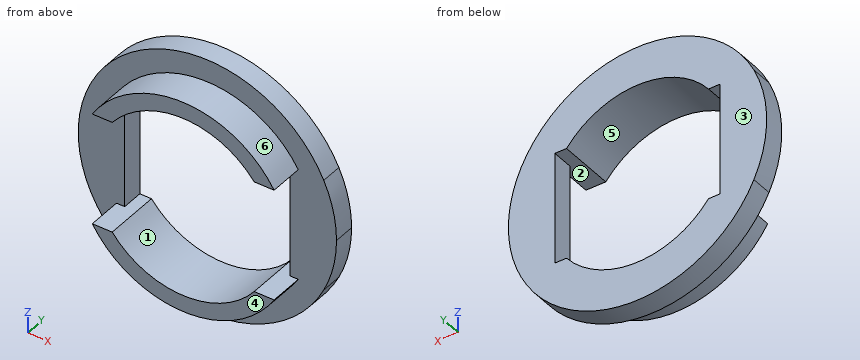
```python
from build123d import *

# Parameters (mm, degrees)
BOSS_EXTRUDE1_DEPTH     = 2.5
BOSS_EXTRUDE2_DEPTH     = 4
CUT_EXTRUDE1_DEPTH      = 5
CUT_EXTRUDE1_DEPTH_BACK = 3.5


with BuildPart() as part:
    # Sketch1 → Boss-Extrude1 (new body)
    with BuildSketch(Plane(origin=(0, 0, 0), x_dir=(1, 0, 0), z_dir=(0, 1, 0))):
        with BuildLine():
            Line((-9.6, -6.5), (-9.6, 6.5))
            Line((-9.6, 6.5), (-13.518505835, 6.5))
            ThreePointArc((-13.518505835, 6.5), (-15, 0), (-13.518505835, -6.5))
            Line((-13.518505835, -6.5), (-9.6, -6.5))
        make_face()
        with BuildLine():
            Line((9.6, -6.5), (-9.6, -6.5))
            Line((-9.6, -6.5), (-13.518505835, -6.5))
            ThreePointArc((-13.518505835, -6.5), (0, -15), (13.518505835, -6.5))
            Line((13.518505835, -6.5), (9.6, -6.5))
        make_face()
        with BuildLine():
            Line((-13.518505835, 6.5), (-9.6, 6.5))
            Line((-9.6, 6.5), (9.6, 6.5))
            Line((9.6, 6.5), (13.518505835, 6.5))
            ThreePointArc((13.518505835, 6.5), (0, 15), (-13.518505835, 6.5))
        make_face()
        with BuildLine():
            Line((13.518505835, 6.5), (9.6, 6.5))
            Line((9.6, 6.5), (9.6, -6.5))
            Line((9.6, -6.5), (13.518505835, -6.5))
            ThreePointArc((13.518505835, -6.5), (14.624937393, -3.333347603), (15, 0))
            ThreePointArc((15, 0), (14.624937393, 3.333347603), (13.518505835, 6.5))
        make_face()
    extrude(amount=BOSS_EXTRUDE1_DEPTH)

    # Sketch2 → Boss-Extrude2 (add)
    with BuildSketch(Plane.XZ):
        with BuildLine():
            ThreePointArc((10.559829544, 6.5), (0, 12.4), (-10.559829544, 6.5))
            Line((-10.559829544, 6.5), (-9.6, 6.5))
            Line((-9.6, 6.5), (-8.246211251, 6.5))
            ThreePointArc((-8.246211251, 6.5), (0, 10.5), (8.246211251, 6.5))
            Line((8.246211251, 6.5), (9.6, 6.5))
            Line((9.6, 6.5), (10.559829544, 6.5))
        make_face()
        with BuildLine():
            Line((-9.6, -6.5), (-10.559829544, -6.5))
            ThreePointArc((-10.559829544, -6.5), (0, -12.4), (10.559829544, -6.5))
            Line((10.559829544, -6.5), (9.6, -6.5))
            Line((9.6, -6.5), (8.246211251, -6.5))
            ThreePointArc((8.246211251, -6.5), (0, -10.5), (-8.246211251, -6.5))
            Line((-8.246211251, -6.5), (-9.6, -6.5))
        make_face()
    extrude(amount=BOSS_EXTRUDE2_DEPTH)

    # Sketch2<3> → Cut-Extrude1 (cut, two sides)
    with BuildSketch(Plane.XZ) as cut_extrude1_sk:
        with BuildLine():
            ThreePointArc((8.246211251, 6.5), (0, 10.5), (-8.246211251, 6.5))
            Line((-8.246211251, 6.5), (8.246211251, 6.5))
        make_face()
        with BuildLine():
            Line((8.246211251, -6.5), (-8.246211251, -6.5))
            ThreePointArc((-8.246211251, -6.5), (0, -10.5), (8.246211251, -6.5))
        make_face()
    extrude(amount=CUT_EXTRUDE1_DEPTH, mode=Mode.SUBTRACT)
    extrude(cut_extrude1_sk.sketch, amount=-CUT_EXTRUDE1_DEPTH_BACK, mode=Mode.SUBTRACT)


solid = part.part
```
Work out the finished part from the listing and answer in its coordinate system (mm). Face numbers are marked on the shaded views. A direction names the side the tool comes from. Coordinates: 2 decimals unless noted, no trailing zeros. Loops run counter-clockwise (first coordinate to the right, second up) from the corner with the lowest first, then second, coordinate; pieces in that order, holes last. Notation, with made-up numbers: (25, 29) - (58, 29) arc R16 ccw to (58, 35) - close; hole circle Ø2 at (89.25, 49.5). An arc over 180 degrees is marked (long way). Use a Markdown table: item, result.
Item 1: Find section D-D, the plane z = 11. Determine the outline of the cut face in (x, y), and give its area (3 significant figures).
Evaluation:
| item | result |
|---|---|
| outline | (-10.2, 0) - (-5.72, 0) - (-5.72, -4) - (5.72, -4) - (5.72, 0) - (10.2, 0) - (10.2, 2.5) - (-10.2, 2.5) - close |
| area | 96.8 mm2 |
Item 2: Find section B-B, the plane z = -4.5. Determine the outline of the cut face in (x, y), and give its area (3 significant figures).
Evaluation:
| item | result |
|---|---|
| outline | (-14.31, 0) - (-9.6, 0) - (-9.6, 2.5) - (-14.31, 2.5) - close; (9.6, 0) - (14.31, 0) - (14.31, 2.5) - (9.6, 2.5) - close |
| area | 23.5 mm2 |
Item 3: The mould has two halves that part along Z. Classify the marked faces 4, 5 and 6: +Z half, -Z half, draft (parallel to the pull), parting line (faces both ways), or undercut.
Evaluation:
| item | result |
|---|---|
| face 4 | draft |
| face 5 | undercut |
| face 6 | +Z half |
Item 4: Find section C-C, the plane x = -4. Determine the outline of the cut face in (y, z).
Evaluation:
| item | result |
|---|---|
| outline | (-4, -11.74) - (0, -11.74) - (0, -14.46) - (2.5, -14.46) - (2.5, -9.71) - (-4, -9.71) - close; (-4, 9.71) - (2.5, 9.71) - (2.5, 14.46) - (0, 14.46) - (0, 11.74) - (-4, 11.74) - close |
Item 5: For the marked faces 1, 2 and 3, determine the directions among +Z, -Z, +X, -X, +Y, -Y from which every point of the face is accessible in a straight line to the end or side of a thin tool.
Evaluation:
| item | result |
|---|---|
| face 1 | +Y, -Y |
| face 2 | -Y |
| face 3 | +Z, -Z, +X, -X, +Y |
Item 6: Consider probe 1 along Z at (x, y) = (-0.25, -2); probe 2 along Y at (x, z) = (11.75, -3); probe 3 along Z at (x, y) = (6.75, -3). Determine where each line is inside the solid, lowest interval first. Write a range as from..to.
Evaluation:
| item | result |
|---|---|
| probe 1 | z = -12.4..-10.5, 10.5..12.4 |
| probe 2 | y = 0..2.5 |
| probe 3 | z = -10.4..-8.04, 8.04..10.4 |
Item 7: Given pin 1 Ø2.5 at (x, y) = (9, 0.5) entering from -Z; pin 2 Ø3 at (x, z) = (-9, 9) entering from -Y; pin 3 Ø2.5 at (x, y) = (9, 0.5) entering from +Z; pin 4 Ø2 at (x, y) = (-12, 0) entering from -Z, each flat-ended and moving along its own axis, determine where each tip first touches the part or whether it passes through.
Evaluation:
| item | result |
|---|---|
| pin 1 | stops at z = -12.84 |
| pin 2 | stops at y = -4 |
| pin 3 | stops at z = 12.84 |
| pin 4 | stops at z = -10.2 |
Item 8: Find section A-A, the plane y = -1. Determine the outline of the cut face in (x, z).
Evaluation:
| item | result |
|---|---|
| outline | (-10.56, -6.5) arc R12.4 ccw to (10.56, -6.5) - (8.25, -6.5) arc R10.5 cw to (-8.25, -6.5) - close; (-10.56, 6.5) - (-8.25, 6.5) arc R10.5 cw to (8.25, 6.5) - (10.56, 6.5) arc R12.4 ccw to start |
